```python
from build123d import *

# Parameters (mm, degrees)
BOSS_EXTRUDE1_DEPTH = 9.3
CHAMFER1_SIZE       = 1.2


with BuildPart() as part:
    # Sketch1 → Boss-Extrude1 (new body)
    with BuildSketch(Plane.XY):
        Polygon((9.25, -5.34048999), (9.25, 5.34048999), (0, 10.68097998), (-9.25, 5.34048999), (-9.25, -5.34048999), (0, -10.68097998), align=None)
    extrude(amount=-BOSS_EXTRUDE1_DEPTH)

    # Sketch2 → Revolve1 (revolve)
    with BuildSketch(Plane(origin=(0, 0, 0), x_dir=(0, 0, -1), z_dir=(1, 0, 0))):
        Polygon((9.3, 12.25), (12.5, 12.25), (12.5, 6.35), (41, 6.35), (41, 0), (9.3, 0), align=None)
    revolve(axis=Axis((0, 0, -41), (0, 0, 1)))

    # Sketch3 → Cut-Revolve1 (revolve, cut)
    with BuildSketch(Plane(origin=(0, 0, 0), x_dir=(0, 0, -1), z_dir=(1, 0, 0)), mode=Mode.PRIVATE) as cut_revolve1_sk:
        Polygon((0, 8.68097998), (2, 10.68097998), (0, 10.68097998), align=None)
    revolve(cut_revolve1_sk.sketch.rotate(Axis((0, 0, 0), (0, 0, -1)), 300.000000037), axis=Axis((0, 0, 0), (0, 0, -1)), mode=Mode.SUBTRACT)

    # Chamfer1
    chamfer1_edges = [part.edges().sort_by_distance(p)[0] for p in [
        (0, -6.35, -41),
    ]]
    chamfer(chamfer1_edges, length=CHAMFER1_SIZE)


solid = part.part
```
Design review of the part built by this model. Coordinates are the model's own, in mm. A direction names the side the tool comes from. Coordinates: 2 decimals unless noted, no trailing zeros. Order: outer loops, then holes, each group sorted by start corner. A loop starts at its lowest first (then second) coordinate and runs counter-clockwise, first axis right, second up. Notation, with made-up numbers: M 37.5,83.5 L 80.5,83.5 A18 cw 80.5,116.5 Z; hole C 31,-31 d7. An arc over 180 degrees is marked long. Answer as a JSON object with one key per item and string values. Group by question number.
1) Add section C-C, the plane x = -10.25. Write out the cut boundary in (y, z), then the cut area to 3 significant figures.
2) Add section A-A, the plane y = 0. Write out the cut boundary in (x, z).
3) Add section B-B, the plane z = -35. Write out the cut boundary in (x, y), then the cut area to 3 significant figures.
4) Wall thickness on L1, parallel to Z at x = 11, y = 2.5; L2, parallel to X at y = -5.25, z = -5.5; L3, parallel to Z at x = -4.25, y = -7.25: over which ranges is each line inside the solid? List them lowest first.
5) For pin 1 (6 mm diameter, centred on y = -6, z = -17.5, fed in from -X); pin 2 (6 mm diameter, centred on x = 4.5, z = -24.5, fed in from -Y); pin 3 (3 mm diameter, centred on x = -2, z = -27, fed in from -Y), all flat-tipped, find the tip position at first contact; note any pin that passes through.
6) Tool access review of faces 1 (the flat face through (-4.56, 8.05, -4.87)), 2 (the flat face through (5, 5, -12.5)), 3 (the flat face through (9.25, 0, -5)): name each direction out of +Z, -Z, +X, -X, +Y, -Y from which nothing blocks a thin tool from reaching the whole face with its end or side.
Computed values:
{
 "1": {"outline": "M -6.71,-12.5 L 6.71,-12.5 L 6.71,-9.3 L -6.71,-9.3 Z", "area": "42.9 mm^2"},
 "2": {"outline": "M -12.25,-12.5 L -6.35,-12.5 L -6.35,-39.8 L -5.15,-41 L 5.15,-41 L 6.35,-39.8 L 6.35,-12.5 L 12.25,-12.5 L 12.25,-9.3 L 9.25,-9.3 L 9.25,-0.57 L 8.68,0 L -8.68,0 L -9.25,-0.57 L -9.25,-9.3 L -12.25,-9.3 Z"},
 "3": {"outline": "C 0,0 d12.7", "area": "127 mm^2"},
 "4": {"L1": "z = -12.5 to -9.3", "L2": "x = -9.25 to 9.25", "L3": "z = -12.5 to 0"},
 "5": {"pin 1": "stops at x = -5.6", "pin 2": "stops at y = -6.17", "pin 3": "stops at y = -6.33"},
 "6": {"face 1": "+Z, -X, +Y", "face 2": "-Z", "face 3": "+Z, +X, +Y, -Y"}
}
